Geometry: see drawing. Coordinates: mm, zero at the bounding-box minimum. A direction names the side the tool comes from. Round coordinates to 2 decimals unless told otherwise and drop trailing zeros. Write each loop counter-clockwise with the first axis right and the second up, starting at its lowest first coordinate (ties: lowest second). Pieces come first, ordered by that corner, then holes. Notation, with made-up numbers: (74, 87.25) -> (82, 87.25) arc R27 ccw to (82, 103.25) -> close; hole circle Ø1 at (40, -3.5). An arc over 180 degrees is marked (long way). Write item = value, one per line.
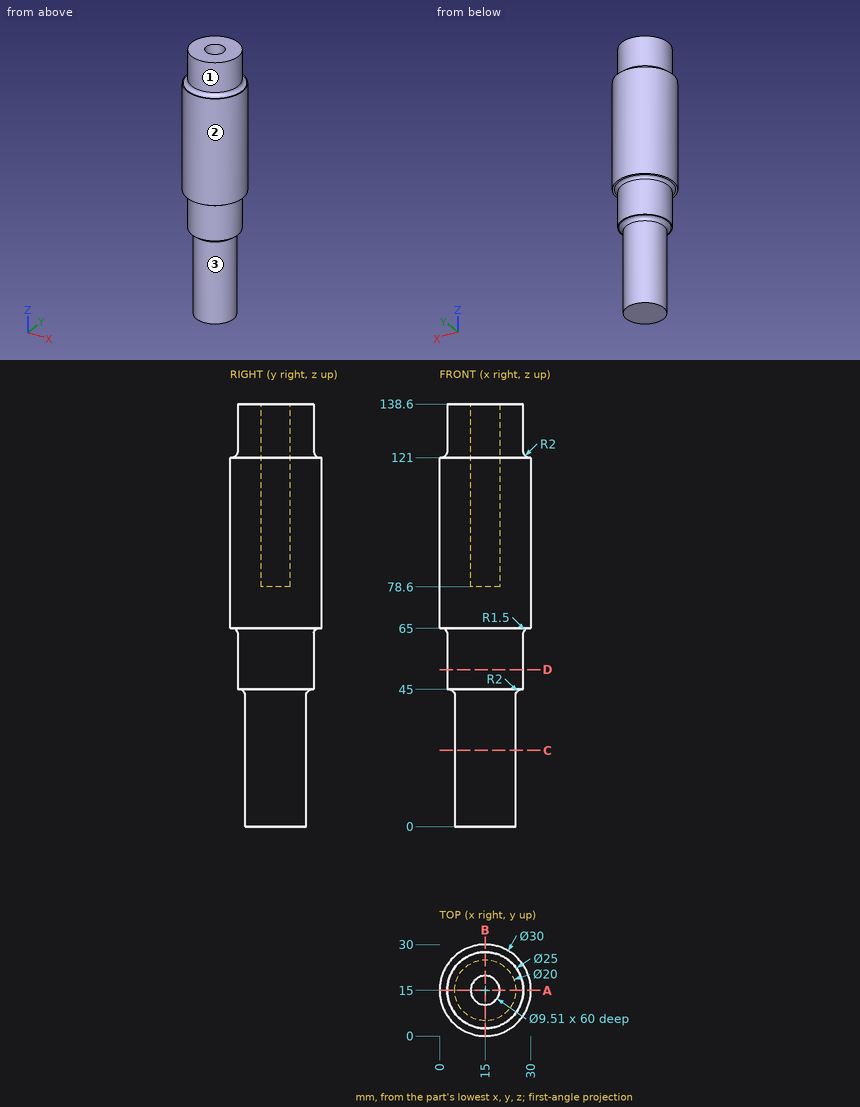
1) Line query: L1, parallel to Y at x = 15, z = 125 (3 decimals); L2, parallel to Y at x = 15, z = 92.5 (3 decimals); L3, parallel to X at y = 13.5, z = 122. Output: solid intervals per line, ascending. Write a range as from..to.
Solutions:
L1 = 2.5..10.245, 19.755..27.5
L2 = 0..10.245, 19.755..30
L3 = 2.32..10.49, 19.51..27.68
2) Cut plane D-D (z = 51.5). Return the cut outline in (x, y), and give its area (3 significant figures).
Solutions:
outline = circle Ø25 at (15, 15)
area = 491 mm^2
3) Cut plane A-A (y = 15). Return the cut outline in (x, z) (3 decimals), and give its area (3 significant figures).
Solutions:
outline = (0, 65) -> (1, 65) arc R1.5 cw to (2.5, 63.5) -> (2.5, 45) -> (3, 45) arc R2 cw to (5, 43) -> (5, 0) -> (25, 0) -> (25, 43) arc R2 cw to (27, 45) -> (27.5, 45) -> (27.5, 63.5) arc R1.5 cw to (29, 65) -> (30, 65) -> (30, 121) -> (29.5, 121) arc R2 cw to (27.5, 123) -> (27.5, 138.6) -> (19.755, 138.6) -> (19.755, 78.6) -> (10.245, 78.6) -> (10.245, 138.6) -> (2.5, 138.6) -> (2.5, 123) arc R2 cw to (0.5, 121) -> (0, 121) -> close
area = 2,950 mm^2
4) Cut plane C-C (z = 25). Return the cut outline in (x, y).
Solutions:
outline = circle Ø20 at (15, 15)
5) First-contact query: P1, Ø12, axis at y = 10.5, z = 55, coming from the -X side; P2, Ø3, axis at x = 19.5, z = 67, coming from the +Y side; P3, Ø4, axis at x = 16, z = 41.5, coming from the +Y side; P4, Ø12.5, axis at x = 17.5, y = 21, coming from the -Z side. Flat tips, straight axial feed; report the tip coordinate or a pass-through.
Solutions:
P1 = 2.5
P2 = 29.7
P3 = 25.04
P4 = 0
6) Access query for the marked faces 1, 2 and 3. Directions: +Z, -Z, +X, -X, +Y, -Y. A direction counts if a zero-diameter tool reaches every point of the face in a straight line with its end or side. Return the directions, or none.
Solutions:
face_1 = +Z
face_2 = +Z, -Z
face_3 = -Z
